The figure shows three views and two pictorial views of one solid part (mm, origin at its lowest corner). Answer the questions. Give positions to 0.01 mm unless a question says otherwise; leave off trailing zeros. Write each loop counter-clockwise with the first axis right and the second up, starting at its lowest first coordinate (ties: lowest second). Pieces come first, ordered by that corner, then holes. Notation, with made-up numbers: (56, 6.5) - (109, 6.5) arc R24 cw to (109, 40.5) - close; hole circle Ø11 at (75, 18). An arc over 180 degrees is marked (long way). Answer as CSV lines item,"result". Start each with the question number.
(1) Each of these flat-tipped pins is pushed along its axis until it touches: pin 1 Ø1.5 at (x, z) = (67, 1) entering from +Y; pin 2 Ø3.5 at (x, y) = (102.5, 70) entering from -Z; pin 3 Ø1 at (x, z) = (81, 0.5) entering from -Y. Where does it stop, or does it pass through?
(2) For a pull along Z with two mould halves and no side action, classify the marked faces 1 and 2 as pulls with the +Z half, pulls with the -Z half, needs draft (parallel to the pull), parting line crosses it, or undercut.
(3) Find section B-B (y = 37.5). Write down the section's boundary in (x, z), then the cut area to 3 significant figures.
(4) Find section A-A (x = 70). Write down the section's boundary in (y, z), then the cut area to 3 significant figures.
(5) Straight lines are drawn through the part: probe 1 along Y at (x, z) = (69, 1.65); probe 2 along X at (y, z) = (92, 2.9); probe 3 along Y at (x, z) = (74, 2.4). For each, find the intervals that lie inside material, in ascending order.
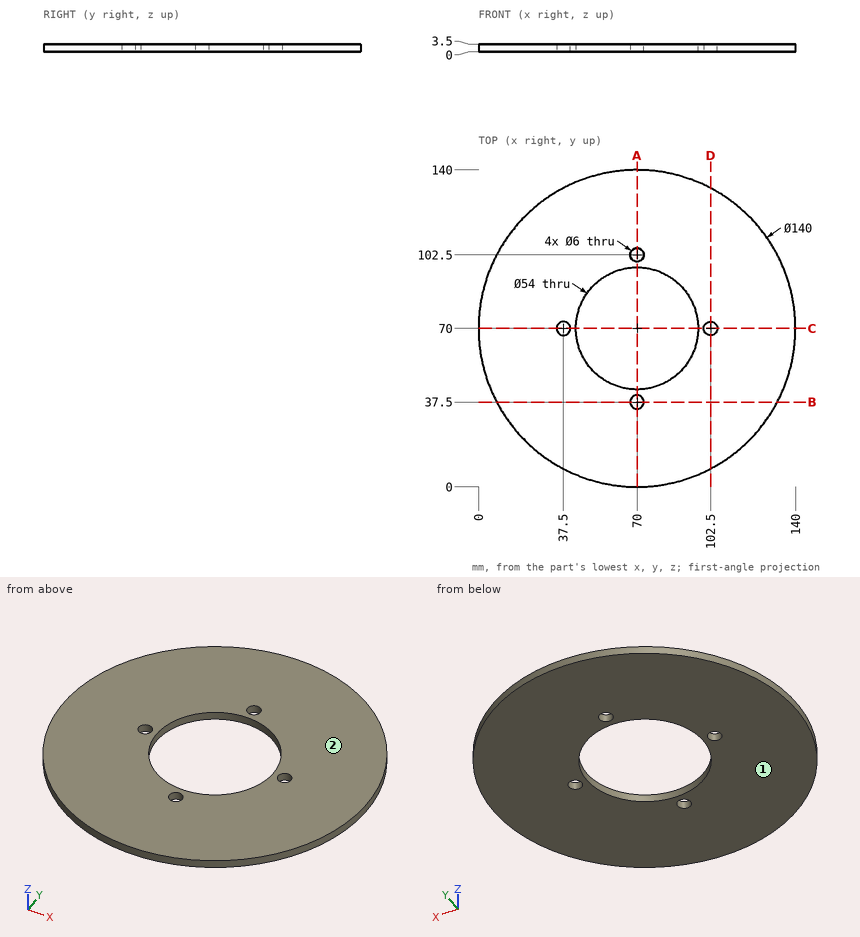
Result set:
1,pin 1,"y = 139.96"
1,pin 2,"through"
1,pin 3,"y = 0.79"
2,face 1,"pulls with the -Z half"
2,face 2,"pulls with the +Z half"
3,outline,"(8, 0) - (67, 0) - (67, 3.5) - (8, 3.5) - close; (73, 0) - (132, 0) - (132, 3.5) - (73, 3.5) - close"
3,area,"413 mm^2"
4,outline,"(0, 0) - (34.5, 0) - (34.5, 3.5) - (0, 3.5) - close; (40.5, 0) - (43, 0) - (43, 3.5) - (40.5, 3.5) - close; (97, 0) - (99.5, 0) - (99.5, 3.5) - (97, 3.5) - close; (105.5, 0) - (140, 0) - (140, 3.5) - (105.5, 3.5) - close"
4,area,"259 mm^2"
5,probe 1,"0.01 to 34.67, 40.33 to 43.02, 96.98 to 99.67, 105.33 to 139.99"
5,probe 2,"3.55 to 54.35, 85.65 to 136.45"
5,probe 3,"0.11 to 43.3, 96.7 to 139.89"
